Verification items for the finished model (mm, model axes). Face numbers are marked on the shaded views. A direction names the side the tool comes from. Give positions to 0.01 mm unless a question says otherwise; leave off trailing zeros. Loops run counter-clockwise (first coordinate to the right, second up) from the corner with the lowest first, then second, coordinate; pieces in that order, holes last. Notation, with made-up numbers: M -39.5,17.25 L -2.5,17.25 A15 cw -2.5,29.25 Z; hole C -17.5,-35 d3. An arc over 180 degrees is marked long. Answer in a Markdown table with one row per item.
```python
from build123d import *

# Parameters (mm, degrees)
F0_R     = 3
F0_R_2   = 2.25
F1_DEPTH = 1.5
F2_DEPTH = 4
F3_R     = 0.5


with BuildPart() as f1:
    # F0 (on Top) → F1 (new body)
    with BuildSketch(Plane.XY):
        Circle(F0_R)
        Circle(F0_R_2, mode=Mode.SUBTRACT)
        Circle(F0_R_2)
    extrude(amount=F1_DEPTH)

    # F0 (on Top) → F2 (join)
    with BuildSketch(Plane.XY):
        Circle(F0_R_2)
    extrude(amount=F2_DEPTH)

    # F3
    f3_edges = [f1.edges().sort_by_distance(p)[0] for p in [
        (-2.25, 0, 4),
    ]]
    fillet(f3_edges, radius=F3_R)


solid = f1.part
```
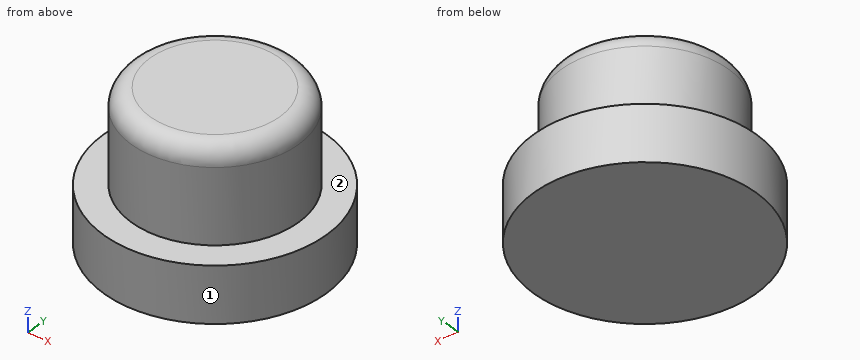
Item 1: Tool access check on the marked faces 1 and 2. Record the directions out of +Z, -Z, +X, -X, +Y, -Y that give a thin tool (end or side, any length) a straight path to the whole face; none if there is none.
Reported:
| item | result |
|---|---|
| face 1 | +Z, -Z |
| face 2 | +Z |
Item 2: Sectioned sample at A-A (x = 0). Record the cut outline in (y, z).
Reported:
| item | result |
|---|---|
| outline | M -3,0 L 3,0 L 3,1.5 L 2.25,1.5 L 2.25,3.5 A0.5 ccw 1.75,4 L -1.75,4 A0.5 ccw -2.25,3.5 L -2.25,1.5 L -3,1.5 Z |
Item 3: Go/stop test with a flat-tipped pin: pin 1 (3 mm diameter, centred on x = 1, y = 2, fed in from -Z). Record where the tip stops, or that it passes through.
Reported:
| item | result |
|---|---|
| pin 1 | stops at z = 0 |
Item 4: Scan lines: L1, parallel to Y at x = -0.05, z = 3.5; L2, parallel to Z at x = -1.5, y = -2.05. Record each from-to range of solid material in increasing order. Write a range as [from, to].
Reported:
| item | result |
|---|---|
| L1 | y = [-2.25, 2.25] |
| L2 | z = [0, 1.5] |
Item 5: Sectioned sample at C-C (z = 0.7). Record the cut outline in (x, y), and give its area (3 significant figures).
Reported:
| item | result |
|---|---|
| outline | C 0,0 d6 |
| area | 28.3 mm^2 |
Item 6: Sectioned sample at D-D (z = 2.25). Record the cut outline in (x, y).
Reported:
| item | result |
|---|---|
| outline | C 0,0 d4.5 |
